Can you work these out from the drawing? Everything is in mm from the part's minimum corner. A direction names the side the tool comes from. Coordinates: 2 decimals unless noted, no trailing zeros. Order: outer loops, then holes, each group sorted by start corner. A loop starts at its lowest first (then second) coordinate and runs counter-clockwise, first axis right, second up. Notation, with made-up numbers: (43, 85) -> (79, 85) arc R25 ccw to (79, 107) -> close; hole circle Ø8 at (75, 76.5). An arc over 180 degrees is marked (long way). Answer in a Markdown table with one row per item.
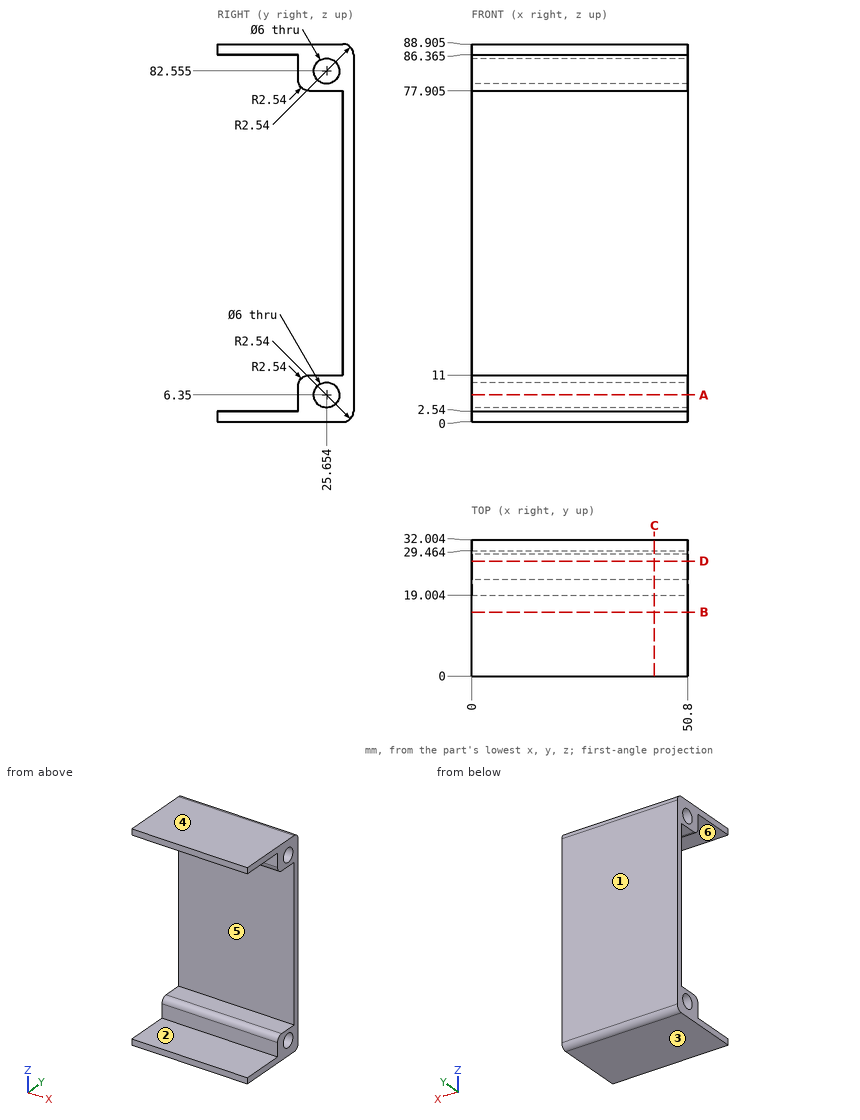
(1) On a 3-axis mill with a long thin cutter (end or side, diameter ignored), from which of +Z, -Z, +X, -X, +Y, -Y can I reach the whole of each face in a straight line? I mean the marked faces 1 and 2. Say none if no direction works.
Response values:
| item | result |
|---|---|
| face 1 | +Z, -Z, +X, -X, +Y |
| face 2 | +X, -X, -Y |
(2) Suppose I cut it at D-D (y = 27). Please give me the cut outline in (x, z) (3 decimals), and give its area (3 significant figures).
Response values:
| item | result |
|---|---|
| outline | (0, 0) -> (50.8, 0) -> (50.8, 3.669) -> (0, 3.669) -> close; (0, 9.031) -> (50.8, 9.031) -> (50.8, 11) -> (0, 11) -> close; (0, 77.905) -> (50.8, 77.905) -> (50.8, 79.874) -> (0, 79.874) -> close; (0, 85.236) -> (50.8, 85.236) -> (50.8, 88.905) -> (0, 88.905) -> close |
| area | 573 mm2 |
(3) Suppose I cut it at B-B (y = 15). Please give me the cut outline in (x, z) (3 decimals).
Response values:
| item | result |
|---|---|
| outline | (0, 0) -> (50.8, 0) -> (50.8, 2.54) -> (0, 2.54) -> close; (0, 86.365) -> (50.8, 86.365) -> (50.8, 88.905) -> (0, 88.905) -> close |
(4) Suppose I cut it at C-C (x = 43). Please give me the cut outline in (y, z) (3 decimals), and give its area (3 significant figures).
Response values:
| item | result |
|---|---|
| outline | (0, 0) -> (29.464, 0) arc R2.54 ccw to (32.004, 2.54) -> (32.004, 86.365) arc R2.54 ccw to (29.464, 88.905) -> (0, 88.905) -> (0, 86.365) -> (19.004, 86.365) -> (19.004, 80.445) arc R2.54 ccw to (21.544, 77.905) -> (29.464, 77.905) -> (29.464, 11) -> (21.544, 11) arc R2.54 ccw to (19.004, 8.46) -> (19.004, 2.54) -> (0, 2.54) -> close; hole circle Ø6 at (25.654, 6.35); hole circle Ø6 at (25.654, 82.555) |
| area | 490 mm2 |
(5) Will these pins go through, and if not, where does the flat tip stop? pin 1 Ø1.5 at (x, z) = (6, 26.5) entering from -Y; pin 2 Ø1.8 at (x, z) = (34, 83) entering from -Y.
Response values:
| item | result |
|---|---|
| pin 1 | y = 29.46 |
| pin 2 | y = 19 |
(6) We'd pull the mould along Z, two halves only. Please class the marked faces 3, 4, 5 and 6: +Z half, -Z half, draft (parallel to the pull), parting line (faces both ways), or undercut.
Response values:
| item | result |
|---|---|
| face 3 | -Z half |
| face 4 | +Z half |
| face 5 | undercut |
| face 6 | undercut |
(7) I need wall thicknesses on line 1 (Y direction, x = 25, z = 6.35); line 2 (Z direction, x = 44, y = 22) (3 decimals); line 3 (Z direction, x = 19, y = 26) (3 decimals). Which ranges of each line are inside material? Lowest first, please. Write a range as [from, to].
Response values:
| item | result |
|---|---|
| line 1 | [19, 22.65], [28.65, 32] |
| line 2 | [0, 11], [77.905, 88.905] |
| line 3 | [0, 3.37], [9.33, 11], [77.905, 79.575], [85.535, 88.905] |
(8) Suppose I cut it at A-A (z = 6.35). Please give me the cut outline in (x, y), and give its area (3 significant figures).
Response values:
| item | result |
|---|---|
| outline | (0, 19) -> (50.8, 19) -> (50.8, 22.65) -> (0, 22.65) -> close; (0, 28.65) -> (50.8, 28.65) -> (50.8, 32) -> (0, 32) -> close |
| area | 356 mm2 |
